from build123d import *

# Parameters (mm, degrees)
BOSS_EXTRUDE1_DEPTH     = 40
SKETCH2_R               = 24
BOSS_EXTRUDE2_DEPTH     = 40
SKETCH3_R               = 24
BOSS_EXTRUDE3_DEPTH     = 40
SCALE1_SCALE            = 0.125
FILLET3_R               = 4
FILLET4_R               = 4
CUT_EXTRUDE1_DEPTH      = 38.275
CUT_EXTRUDE1_DEPTH_BACK = 6
SKETCH5_OUTSIDE_W       = 249.408
SKETCH5_OUTSIDE_H       = 169.408
CUT_EXTRUDE2_DEPTH      = 38.275
CUT_EXTRUDE2_DEPTH_BACK = 6
SKETCH7_R               = 1.5
CUT_EXTRUDE3_DEPTH      = 5


with BuildPart() as part:
    # Sketch1 → Boss-Extrude1 (new body)
    with BuildSketch(Plane(origin=(0, 0, 0), x_dir=(1, 0, 0), z_dir=(0, 1, 0))):
        Polygon((-173.422280891, 480), (-173.422280891, 450), (-800, 450), (-800, -450), (-173.422280891, -450), (-173.422280891, -480), (800, -480), (800, 480), align=None)
    extrude(amount=-BOSS_EXTRUDE1_DEPTH)

    # Sketch2 → Boss-Extrude2 (add)
    with BuildSketch(Plane.XY.offset(480)):
        with BuildLine():
            Line((218, 0), (298, 0))
            Line((298, 0), (298, 100))
            ThreePointArc((298, 100), (258, 140), (218, 100))
            Line((218, 100), (218, 0))
        make_face()
        with Locations((258, 100)):
            Circle(SKETCH2_R, mode=Mode.SUBTRACT)
        with BuildLine():
            Line((650, 258.2), (650, 0))
            Line((650, 0), (730, 0))
            Line((730, 0), (730, 258.2))
            ThreePointArc((730, 258.2), (690, 298.2), (650, 258.2))
        make_face()
        with Locations((690, 258.2)):
            Circle(SKETCH2_R, mode=Mode.SUBTRACT)
        Polygon((650, 0), (298, 0), (218, 0), (-173.422280891, 0), (-173.422280891, -40), (800, -40), (800, 0), (730, 0), align=None)
    extrude(amount=-BOSS_EXTRUDE2_DEPTH)

    # Mirror1: part across plane


with BuildPart() as part_1:
    add(part.part)
    add(part.part.mirror(Plane.XY))

    # Sketch3 → Boss-Extrude3 (add)
    with BuildSketch(Plane.XY.offset(450)):
        with BuildLine():
            Line((-414, 0), (-334, 0))
            Line((-334, 0), (-334, 162.7))
            ThreePointArc((-334, 162.7), (-374, 202.7), (-414, 162.7))
            Line((-414, 162.7), (-414, 0))
        make_face()
        with Locations((-374, 162.7)):
            Circle(SKETCH3_R, mode=Mode.SUBTRACT)
        with BuildLine():
            Line((-264, 0), (-184, 0))
            Line((-184, 0), (-184, 162.7))
            ThreePointArc((-184, 162.7), (-224, 202.7), (-264, 162.7))
            Line((-264, 162.7), (-264, 0))
        make_face()
        with Locations((-224, 162.7)):
            Circle(SKETCH3_R, mode=Mode.SUBTRACT)
    boss_extrude3 = extrude(amount=-BOSS_EXTRUDE3_DEPTH)

    # Mirror2: Boss-Extrude3 across plane
    add(boss_extrude3.mirror(Plane.XY))


with BuildPart() as part_2:
    # Scale1: scaled about (22.22402446, -11.339866564, 0)
    add(part_1.part.scale(SCALE1_SCALE).moved(Location((19.446021402, -9.922383243, 0))))

    # Fillet3
    fillet3_edges = [part_2.edges().sort_by_distance(p)[0] for p in [
        (-32.303978598, -9.922383243, 53.75),
        (-13.553978598, -9.922383243, 53.75),
        (-32.303978598, -9.922383243, -53.75),
        (-13.553978598, -9.922383243, -53.75),
        (46.696021403, -9.922383243, 57.5),
        (100.696021403, -9.922383243, 57.5),
        (100.696021403, -9.922383243, -57.5),
        (46.696021403, -9.922383243, -57.5),
    ]]
    fillet(fillet3_edges, radius=FILLET3_R)

    # Fillet4
    fillet4_edges = [part_2.edges().sort_by_distance(p)[0] for p in [
        (-3.553978598, -9.922383243, -53.75),
        (-22.303978598, -9.922383243, -53.75),
        (56.696021403, -9.922383243, -57.5),
        (110.696021402, -9.922383243, -57.5),
        (110.696021402, -9.922383243, 57.5),
        (56.696021403, -9.922383243, 57.5),
        (-3.553978598, -9.922383243, 53.75),
        (-22.303978598, -9.922383243, 53.75),
    ]]
    fillet(fillet4_edges, radius=FILLET4_R)

    # Sketch4 → Cut-Extrude1 (cut, two sides)
    with BuildSketch(Plane(origin=(0, -9.922383244, 0), x_dir=(1, 0, 0), z_dir=(0, 1, 0))) as cut_extrude1_sk:
        with BuildLine():
            Line((-60.553978598, 45), (99.446021402, 45))
            ThreePointArc((99.446021402, 45), (106.517089214, 42.071067812), (109.446021402, 35))
            Line((109.446021402, 35), (109.446021402, -35))
            ThreePointArc((109.446021402, -35), (106.517089214, -42.071067812), (99.446021402, -45))
            Line((99.446021402, -45), (-60.553978598, -45))
            ThreePointArc((-60.553978598, -45), (-67.62504641, -42.071067812), (-70.553978598, -35))
            Line((-70.553978598, -35), (-70.553978598, 35))
            ThreePointArc((-70.553978598, 35), (-67.62504641, 42.071067812), (-60.553978598, 45))
        make_face()
    extrude(amount=CUT_EXTRUDE1_DEPTH, mode=Mode.SUBTRACT)
    extrude(cut_extrude1_sk.sketch, amount=-CUT_EXTRUDE1_DEPTH_BACK, mode=Mode.SUBTRACT)

    # Sketch5 outside → Cut-Extrude2 (cut, two sides)
    with BuildSketch(Plane(origin=(0, -9.922383244, 0), x_dir=(1, 0, 0), z_dir=(0, 1, 0))) as cut_extrude2_sk:
        with Locations((19.446, 0)):
            Rectangle(SKETCH5_OUTSIDE_W, SKETCH5_OUTSIDE_H)
        Polygon((0, 0), (123.509842575, 0), (123.509842575, -66.212941814), (-94.641009198, -66.212941814), (-94.641009198, 0), align=None, mode=Mode.SUBTRACT)
    extrude(amount=CUT_EXTRUDE2_DEPTH, mode=Mode.SUBTRACT)
    extrude(cut_extrude2_sk.sketch, amount=-CUT_EXTRUDE2_DEPTH_BACK, mode=Mode.SUBTRACT)

    # Sketch7 → Cut-Extrude3 (cut)
    with BuildSketch(Plane(origin=(0, 0, 0), x_dir=(-1, 0, 0), z_dir=(0, 0, -1))):
        with Locations((-114.446021402, -12.422383244)):
            Circle(SKETCH7_R)
        with Locations((75.553978598, -12.422383244)):
            Circle(SKETCH7_R)
    extrude(amount=-CUT_EXTRUDE3_DEPTH, mode=Mode.SUBTRACT)


solid = part_2.part
The model under review builds one solid part; all positions refer to its coordinate system, in mm. A direction names the side the tool comes from. Round coordinates to 2 decimals unless told otherwise and drop trailing zeros. Write each loop counter-clockwise with the first axis right and the second up, starting at its lowest first coordinate (ties: lowest second). Pieces come first, ordered by that corner, then holes. Notation, with made-up numbers: (64, 68) - (99, 68) arc R14 cw to (99, 90) - close; hole circle Ø6 at (28, -32.75). An arc over 180 degrees is marked (long way). One line per item, written item: value. Start each with the question number.
1. Consider section B-B on x = -9. Write out the cut boundary in (y, z).
2. Consider section D-D on x = 72. Write out the cut boundary in (y, z), and give its area (3 significant figures).
3. Consider section A-A on z = 7. Write out the cut boundary in (x, y), and give its area (4 significant figures).
4. Clearance check with flat-ended pins moving along their axes: P1, Ø4, axis at y = -0.5, z = 54.5, coming from the +X side; P2, Ø12, axis at x = -6, y = 3, coming from the +Z side; P3, Ø20, axis at x = -10.5, y = 6, coming from the -Z side. State where each tip first meets the part, or that it passes through.
5. Machinability: for faces 1 (the face through (110.696, 8, 58)), 2 (the face through (99.493, -8.782, 57.465)), 3 (the face through (-27, 0, 51.25)), which of the approach directions +Z, -Z, +X, -X, +Y, -Y give a long, thin tool a straight path to every point of the face, cutting with its end or side? Answer none if there is none.
6. To check wall thickness, follow L1, parallel to Z at x = 90, y = -10; L2, parallel to Y at x = 65, z = 55; L3, parallel to Z at x = -5, y = -10.5. State the ranges of each line that lie inside material, in increasing order. Write a range as from..to.
7. The part is to be moulded in two halves that separate along Y. For faces 4 (the face through (72, -11, 60)), 5 (the face through (107.31, 24.88, 57.54)), 6 (the face through (45.493, -8.782, 57.465)), say which applies: released by +Y, released by -Y, zero draft, split by the parting line, or undercut.
8. Consider section C-C on z = 38. Write out the cut boundary in (x, y), and give its area (3 significant figures).
Checks:
1. outline: (-14.92, 45) - (-9.92, 45) - (-9.92, 51.25) - (7.45, 51.25) - (7.45, 56.25) - (-14.92, 56.25) - close; (13.38, 51.25) - (15.4, 51.25) - (15.4, 56.25) - (13.38, 56.25) - close
2. outline: (-14.92, 45) - (-9.92, 45) - (-9.92, 60) - (-14.92, 60) - close
2. area: 75.0 mm^2
3. outline: (-80.55, -14.92) - (-70.55, -14.92) - (-70.55, -9.92) - (-80.55, -9.92) - close; (109.45, -14.92) - (119.45, -14.92) - (119.45, -9.92) - (109.45, -9.92) - close
3. area: 100.0 mm^2
4. P1: stops at x = 110.7
4. P2: stops at z = 56.25
4. P3: stops at z = 51.25
5. face 1: +Z, -Z, +X, +Y
5. face 2: +Z, -Z, +Y
5. face 3: -Z, +X, -X, +Y
6. L1: z = 45..60
6. L2: y = -14.92..-9.92
6. L3: z = 45..56.25
7. face 4: zero draft
7. face 5: undercut
7. face 6: released by +Y
8. outline: (-80.55, -14.92) - (-70.09, -14.92) - (-70.09, -9.92) - (-80.55, -9.92) - close; (108.99, -14.92) - (119.45, -14.92) - (119.45, -9.92) - (108.99, -9.92) - close
8. area: 105 mm^2
